```python
from build123d import *

# Parameters (mm, degrees)
SKETCH2_R           = 2.2479
BOSS_EXTRUDE3_DEPTH = 6.35
SKETCH2_5_W         = 34.29
SKETCH2_5_H         = 3.175
SKETCH2_5_H_2       = 8.89
BOSS_EXTRUDE4_DEPTH = 12.4714
SKETCH3_W           = 16.74
SKETCH3_H           = 8.89
BOSS_EXTRUDE5_DEPTH = 10.414


with BuildPart() as part:
    # Sketch2 → Boss-Extrude3 (new body)
    with BuildSketch(Plane(origin=(0, 0, 0), x_dir=(0, 0, -1), z_dir=(1, 0, 0))):
        Polygon((16.17094154, 0), (8.480621378, 0), (8.480621378, -8.89), (57.15, -8.89), (57.15, 0), (176.670010733, 0), (176.670010733, 89.2048), (49.670010733, 89.2048), (0, 60.116195388), (16.17094154, 30.058097694), align=None)
        with Locations((90.119204984, 82.8548)):
            Circle(SKETCH2_R, mode=Mode.SUBTRACT)
        with Locations((71.642065552, 34.29)):
            Circle(SKETCH2_R, mode=Mode.SUBTRACT)
        with Locations((100.543356523, 21.1455)):
            Circle(SKETCH2_R, mode=Mode.SUBTRACT)
        with Locations((25.4, 55.3212)):
            Circle(SKETCH2_R, mode=Mode.SUBTRACT)
    extrude(amount=-BOSS_EXTRUDE3_DEPTH)

    # Sketch2_5 → Boss-Extrude4 (add)
    with BuildSketch(Plane(origin=(0, 0, 0), x_dir=(0, 0, -1), z_dir=(1, 0, 0))):
        with Locations((40.005, 1.5875)):
            Rectangle(SKETCH2_5_W, SKETCH2_5_H)
        with Locations((40.005, -4.445)):
            Rectangle(SKETCH2_5_W, SKETCH2_5_H_2)
    extrude(amount=BOSS_EXTRUDE4_DEPTH)

    # Sketch3 → Boss-Extrude5 (add)
    with BuildSketch(Plane(origin=(12.4714, 0, 0), x_dir=(0, 0, -1), z_dir=(1, 0, 0))):
        with Locations((31.23, -4.445)):
            Rectangle(SKETCH3_W, SKETCH3_H)
    extrude(amount=BOSS_EXTRUDE5_DEPTH)


solid = part.part
```
Could you check a few things on this model? Use its own coordinates, in mm. A direction names the side the tool comes from. Give positions to 0.01 mm unless a question says otherwise; leave off trailing zeros. Loops run counter-clockwise (first coordinate to the right, second up) from the corner with the lowest first, then second, coordinate; pieces in that order, holes last. Notation, with made-up numbers: (8.25, 56) -> (21.25, 56) arc R24 cw to (21.25, 84) -> close; hole circle Ø8 at (-5, 84.5). An arc over 180 degrees is marked (long way). Put each result on its own line as item: value.
(1) Imagine slicing it at A-A on z = -25.4. Write out the boundary of the cut face in (x, y) (3 decimals), plus the area to 3 significant figures.
Computed:
outline: (-6.35, -8.89) -> (22.885, -8.89) -> (22.885, 0) -> (12.471, 0) -> (12.471, 3.175) -> (0, 3.175) -> (0, 53.073) -> (-6.35, 53.073) -> close; (-6.35, 57.569) -> (0, 57.569) -> (0, 74.991) -> (-6.35, 74.991) -> close
area: 747 mm^2
(2) Please list where these lines run through material, in increasing order: probe 1 along Y at (x, z) = (8.5, -51) (3 decimals); probe 2 along X at (y, z) = (29.5, -106.5); probe 3 along Y at (x, z) = (-2, -25.4). Write a range as [from, to].
Computed:
probe 1: [-8.89, 3.175]
probe 2: [-6.35, 0]
probe 3: [-8.89, 53.07], [57.57, 74.99]
(3) For faces 5 (the face through (6, 3.175, -40)), 6 (the face through (11, -3, -22.86)), 7 (the face through (-3, 0, -116)), which set-ups out of +Z, -Z, +X, -X, +Y, -Y let a thin tool reach every point of the face, with its end or its side?
Computed:
face 5: +Z, -Z, +X, +Y
face 6: +Z, +X, +Y, -Y
face 7: -Z, +X, -X, -Y
(4) Thinking about a two-plate mould opening in Y: for faces 1 (the face through (-3, 44, -176.67)), 2 (the face through (-3.131, 81.487, -88.335)), 3 (the face through (5, -8.89, -38)), 4 (the face through (-3.13, 45.3, -7.97)), which applies, pulls with the +Y half, pulls with the -Y half, needs draft (parallel to the pull), parting line crosses it, or undercut?
Computed:
face 1: needs draft
face 2: undercut
face 3: pulls with the -Y half
face 4: undercut
(5) Imagine slicing it at D-D on x = 8.75. Write out the boundary of the cut face in (y, z) (3 decimals), plus the area to 3 significant figures.
Computed:
outline: (-8.89, -57.15) -> (3.175, -57.15) -> (3.175, -22.86) -> (-8.89, -22.86) -> close
area: 414 mm^2
(6) Imagine slicing it at C-C on y = 34.29. Write out the boundary of the cut face in (x, z).
Computed:
outline: (-6.35, -176.67) -> (0, -176.67) -> (0, -73.89) -> (-6.35, -73.89) -> close; (-6.35, -69.39) -> (0, -69.39) -> (0, -13.89) -> (-6.35, -13.89) -> close
(7) Imagine slicing it at B-B on x = -4.5. Write out the boundary of the cut face in (y, z), plus the area to 3 significant figures.
Computed:
outline: (-8.89, -57.15) -> (0, -57.15) -> (0, -176.67) -> (89.2, -176.67) -> (89.2, -49.67) -> (60.12, 0) -> (30.06, -16.17) -> (0, -16.17) -> (0, -8.48) -> (-8.89, -8.48) -> close; hole circle Ø4.5 at (21.15, -100.54); hole circle Ø4.5 at (34.29, -71.64); hole circle Ø4.5 at (55.32, -25.4); hole circle Ø4.5 at (82.85, -90.12)
area: 14,700 mm^2
(8) I'm going to push flat-ended pins straight in: pin 1 Ø11.5 at (x, z) = (18, -33.5) entering from +Y (3 decimals); pin 2 Ø6 at (y, z) = (55.32, -25.4) entering from +X; pin 3 Ø3.5 at (x, y) = (7.5, -4.5) entering from +Z; pin 4 Ø12 at (x, z) = (8, -151.5) entering from +Y. Where does each tip first touch, or does it pass through?
Computed:
pin 1: y = 3.175
pin 2: x = 0
pin 3: z = -22.86
pin 4: through
